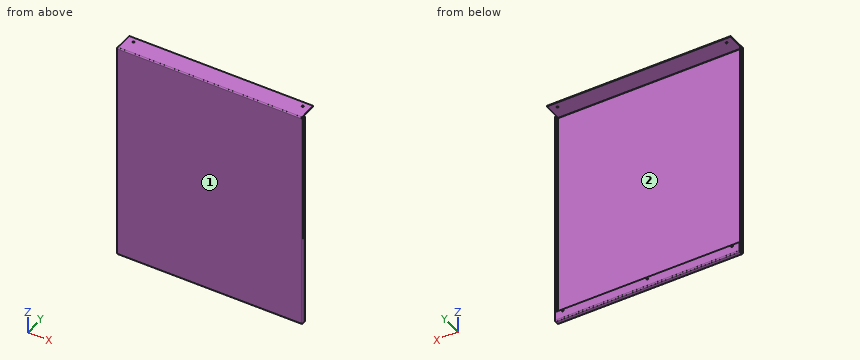
```python
from build123d import *

# Parameters (mm, degrees)
SKETCH1_W                    = 498
SKETCH1_H                    = 604
BASE_FLANGE1_DEPTH           = 2
EDGE_FLANGE1_STRIP_W         = 10
EDGE_FLANGE1_STRIP_H         = 2
EDGE_FLANGE1_STRIP_CUT_DEPTH = 604
EDGE_FLANGE1_DEPTH           = 604
EDGE_FLANGE4_STRIP_W         = 10
EDGE_FLANGE4_STRIP_H         = 2
EDGE_FLANGE4_STRIP_CUT_DEPTH = 497
EDGE_FLANGE4_DEPTH           = 497
EDGE_FLANGE5_STRIP_W         = 10
EDGE_FLANGE5_STRIP_H         = 2
EDGE_FLANGE5_STRIP_CUT_DEPTH = 497
EDGE_FLANGE5_DEPTH           = 497
EDGE_FLANGE6_STRIP_W         = 10
EDGE_FLANGE6_STRIP_H         = 2
EDGE_FLANGE6_STRIP_CUT_DEPTH = 603
EDGE_FLANGE6_DEPTH           = 603
EDGE_FLANGE7_STRIP_W         = 10
EDGE_FLANGE7_STRIP_H         = 2
EDGE_FLANGE7_STRIP_CUT_DEPTH = 496
EDGE_FLANGE7_DEPTH           = 496
SKETCH37_R                   = 2.5
CUT_EXTRUDE2_DEPTH           = 2
SKETCH38_R                   = 2.5
CUT_EXTRUDE3_DEPTH           = 660.824976793
SKETCH39_R                   = 2.5
CUT_EXTRUDE4_DEPTH           = 10


# Sheet-metal steps are written as plain solids
with BuildPart() as part:
    # Sketch1 → Base-Flange1 (new body)
    with BuildSketch(Plane(origin=(0, 0, 0), x_dir=(1, 0, 0), z_dir=(0, 1, 0))):
        Rectangle(SKETCH1_W, SKETCH1_H)
    extrude(amount=BASE_FLANGE1_DEPTH)

    # Edge-Flange1 strip (across the edge) → Edge-Flange1 strip cut (cut)
    with BuildSketch(Plane(origin=(-249, 2, -302), x_dir=(1, 0, 0), z_dir=(0, 0, 1))):
        with Locations((-4, -1)):
            Rectangle(EDGE_FLANGE1_STRIP_W, EDGE_FLANGE1_STRIP_H)
    extrude(amount=EDGE_FLANGE1_STRIP_CUT_DEPTH, mode=Mode.SUBTRACT)

    # Edge-Flange1 section (across the edge) → Edge-Flange1 (add)
    with BuildSketch(Plane(origin=(-249, 2, -302), x_dir=(1, 0, 0), z_dir=(0, 0, 1))):
        with BuildLine():
            Line((-2, 1), (-2, 10))
            Line((-2, 10), (0, 10))
            Line((0, 10), (0, 1))
            ThreePointArc((0, 1), (0.292893219, 0.292893219), (1, 0))
            Line((1, 0), (1, -2))
            ThreePointArc((1, -2), (-1.121320344, -1.121320344), (-2, 1))
        make_face()
    extrude(amount=EDGE_FLANGE1_DEPTH)

    # Edge-Flange4 strip (across the edge) → Edge-Flange4 strip cut (cut)
    with BuildSketch(Plane(origin=(249, 2, -302), x_dir=(0, 0, 1), z_dir=(-1, 0, 0))):
        with Locations((-4, -1)):
            Rectangle(EDGE_FLANGE4_STRIP_W, EDGE_FLANGE4_STRIP_H)
    extrude(amount=EDGE_FLANGE4_STRIP_CUT_DEPTH, mode=Mode.SUBTRACT)

    # Edge-Flange4 section (across the edge) → Edge-Flange4 (add)
    with BuildSketch(Plane(origin=(249, 2, -302), x_dir=(0, 0, 1), z_dir=(-1, 0, 0))):
        with BuildLine():
            Line((-2, 1), (-2, 10))
            Line((-2, 10), (0, 10))
            Line((0, 10), (0, 1))
            ThreePointArc((0, 1), (0.292893219, 0.292893219), (1, 0))
            Line((1, 0), (1, -2))
            ThreePointArc((1, -2), (-1.121320344, -1.121320344), (-2, 1))
        make_face()
    extrude(amount=EDGE_FLANGE4_DEPTH)

    # Edge-Flange5 strip (across the edge) → Edge-Flange5 strip cut (cut)
    with BuildSketch(Plane(origin=(249, 12, -302), x_dir=(0, -1, 0), z_dir=(-1, 0, 0))):
        with Locations((-4, -1)):
            Rectangle(EDGE_FLANGE5_STRIP_W, EDGE_FLANGE5_STRIP_H)
    extrude(amount=EDGE_FLANGE5_STRIP_CUT_DEPTH, mode=Mode.SUBTRACT)

    # Edge-Flange5 section (across the edge) → Edge-Flange5 (add)
    with BuildSketch(Plane(origin=(249, 12, -302), x_dir=(0, -1, 0), z_dir=(-1, 0, 0))):
        with BuildLine():
            Line((-2, 1), (-2, 25))
            Line((-2, 25), (0, 25))
            Line((0, 25), (0, 1))
            ThreePointArc((0, 1), (0.292893219, 0.292893219), (1, 0))
            Line((1, 0), (1, -2))
            ThreePointArc((1, -2), (-1.121320344, -1.121320344), (-2, 1))
        make_face()
    extrude(amount=EDGE_FLANGE5_DEPTH)

    # Edge-Flange6 strip (across the edge) → Edge-Flange6 strip cut (cut)
    with BuildSketch(Plane(origin=(249, 2, 302), x_dir=(-1, 0, 0), z_dir=(0, 0, -1))):
        with Locations((-4, -1)):
            Rectangle(EDGE_FLANGE6_STRIP_W, EDGE_FLANGE6_STRIP_H)
    extrude(amount=EDGE_FLANGE6_STRIP_CUT_DEPTH, mode=Mode.SUBTRACT)

    # Edge-Flange6 section (across the edge) → Edge-Flange6 (add)
    with BuildSketch(Plane(origin=(249, 2, 302), x_dir=(-1, 0, 0), z_dir=(0, 0, -1))):
        with BuildLine():
            Line((-2, 1), (-2, 9))
            Line((-2, 9), (0, 9))
            Line((0, 9), (0, 1))
            ThreePointArc((0, 1), (0.292893219, 0.292893219), (1, 0))
            Line((1, 0), (1, -2))
            ThreePointArc((1, -2), (-1.121320344, -1.121320344), (-2, 1))
        make_face()
    extrude(amount=EDGE_FLANGE6_DEPTH)

    # Edge-Flange7 strip (across the edge) → Edge-Flange7 strip cut (cut)
    with BuildSketch(Plane(origin=(-248, 2, 302), x_dir=(0, 0, -1), z_dir=(1, 0, 0))):
        with Locations((-4, -1)):
            Rectangle(EDGE_FLANGE7_STRIP_W, EDGE_FLANGE7_STRIP_H)
    extrude(amount=EDGE_FLANGE7_STRIP_CUT_DEPTH, mode=Mode.SUBTRACT)

    # Edge-Flange7 section (across the edge) → Edge-Flange7 (add)
    with BuildSketch(Plane(origin=(-248, 2, 302), x_dir=(0, 0, -1), z_dir=(1, 0, 0))):
        with BuildLine():
            Line((-2, 1), (-2, 50))
            Line((-2, 50), (0, 50))
            Line((0, 50), (0, 1))
            ThreePointArc((0, 1), (0.292893219, 0.292893219), (1, 0))
            Line((1, 0), (1, -2))
            ThreePointArc((1, -2), (-1.121320344, -1.121320344), (-2, 1))
        make_face()
    extrude(amount=EDGE_FLANGE7_DEPTH)

    # Sketch37 → Cut-Extrude2 (cut)
    with BuildSketch(Plane(origin=(0, 14, 0), x_dir=(1, 0, 0), z_dir=(0, 1, 0))):
        with Locations(Location((-228.5, 281, 0), (0, 0, 270))):
            Circle(SKETCH37_R)
        with Locations(Location((228.5, 281, 0), (0, 0, 270))):
            Circle(SKETCH37_R)
    extrude(amount=-CUT_EXTRUDE2_DEPTH, mode=Mode.SUBTRACT)

    # Sketch38 → Cut-Extrude3 (cut, through all)
    with BuildSketch(Plane.XY.offset(304)):
        with Locations((228.5, 38)):
            Circle(SKETCH38_R)
        with Locations(Location((-228.5, 38, 0), (0, 0, 270))):
            Circle(SKETCH38_R)
    extrude(amount=-CUT_EXTRUDE3_DEPTH, mode=Mode.SUBTRACT)

    # Sketch39 → Cut-Extrude4 (cut)
    with BuildSketch(Plane(origin=(0, 14, 0), x_dir=(1, 0, 0), z_dir=(0, 1, 0))):
        with Locations(Location((0.468438538, 282, 0), (0, 0, 270))):
            Circle(SKETCH39_R)
    extrude(amount=-CUT_EXTRUDE4_DEPTH, mode=Mode.SUBTRACT)


solid = part.part
```
Design review of the part built by this model. Coordinates are the model's own, in mm. Face numbers are marked on the shaded views. Give positions to 0.01 mm unless a question says otherwise; leave off trailing zeros. Order: outer loops, then holes, each group sorted by start corner. A loop starts at its lowest first (then second) coordinate and runs counter-clockwise, first axis right, second up. Notation, with made-up numbers: M 33.25,67.5 L 46.25,67.5 A19 cw 46.25,87.5 Z; hole C 14,45.25 d5. An arc over 180 degrees is marked long. One line per question, with ' | ' between items. Start each with the question number.
Q1. The part is to be moulded in two halves that separate along X. For the marked faces 1 and 2, say which applies: +X half, -X half, draft (parallel to the pull), parting line (faces both ways), or undercut.
Q2. We need section A-A (x = -37.5). Write out the cut boundary in (y, z), plus the area to 3 significant figures.
Q3. For L1, parallel to X at y = 8, z = 54; L2, parallel to Z at x = 228.5, y = 12.9; L3, parallel to X at y = 13.55, z = -282, list the stretches that pass through material, from the lowest coordinate up. Write a range as [from, to].
Q4. For pin 1 Ø12 at (x, z) = (4.5, -283) entering from +Y; pin 2 Ø0.9 at (x, y) = (249.5, 6) entering from -Z; pin 3 Ø2.5 at (x, y) = (-250, 8.5) entering from -Z, all flat-tipped, find the tip position at first contact; note any pin that passes through.
Q5. We need section B-B (z = -101.5). Write out the cut boundary in (x, y), plus the area to 3 significant figures.
Returned:
1) face 1: draft | face 2: undercut
2) outline: M 0,-301 A3 ccw 3,-304 L 11,-304 A3 ccw 14,-301 L 14,-277 L 12,-277 L 12,-301 A1 cw 11,-302 L 3,-302 A1 cw 2,-301 L 2,301 A1 cw 3,302 L 52,302 L 52,304 L 3,304 A3 ccw 0,301 Z | area: 1,380 mm2
3) L1: [-251, -249], [249, 251] | L2: [-303.32, -283.5], [-278.5, -277], [302, 304] | L3: [-248, -230.79], [-226.21, -2.03], [2.97, 226.21], [230.79, 249]
4) pin 1: y = 14 | pin 2: z = -301 | pin 3: z = -302
5) outline: M -251,3 A3 ccw -248,0 L 248,0 A3 ccw 251,3 L 251,11 L 249,11 L 249,3 A1 cw 248,2 L -248,2 A1 cw -249,3 L -249,12 L -251,12 Z | area: 1,040 mm2
